CAD build for the part. Positions are in the model's coordinates, mm. A direction names the side the tool comes from. Give positions to 0.01 mm unless a question says otherwise; leave off trailing zeros. Loops run counter-clockwise (first coordinate to the right, second up) from the corner with the lowest first, then second, coordinate; pieces in that order, holes last. Notation, with made-up numbers: (-1.75, 24.5) - (19.25, 24.5) arc R32 cw to (19.25, 55.5) - close; hole circle Ø4 at (78, 49). An arc over 180 degrees is marked (long way). Return JSON: item names as keys, results as strings.
Autodesk Inventor part; units mm, degrees
ref_plane "YZ Plane" through (0, 0, 0) normal (1, 0, 0) x (0, 1, 0)
ref_plane "XZ Plane" through (0, 0, 0) normal (0, 1, 0) x (-1, 0, 0)
ref_plane "XY Plane" through (0, 0, 0) normal (0, 0, 1) x (1, 0, 0)
sketch "Sketch1" plane through (0, 0, 0) normal (0, 0, 1) x (1, 0, 0)
  line L0 (0, -9.7468) -> (0, 24.9578) construction
  line L1 (-29.249, 0) -> (29.249, 0) construction
  arc A0 (-18.0821, 3.4154) -> (-16, -4) centre (-16, 0) ccw
  line L2 (-16, -4) -> (16, -4)
  arc A1 (16, -4) -> (18.0821, 3.4154) centre (16, 0) ccw
  line L3 (-18.0821, 3.4154) -> (-4, 12)
  line L4 (-4, 12) -> (-4, 16)
  arc A2 (4, 16) -> (-4, 16) centre (0, 16) ccw
  line L5 (4, 16) -> (4, 12)
  line L6 (4, 12) -> (18.0821, 3.4154)
  point P0 (0, -4)
  dimension "d0" = 40
  dimension "d38" = 8
  dimension "d39" = 24
  dimension "d41" = 4
sketch "Sketch8" plane through (0, 0, 0) normal (0, 0, 1) x (1, 0, 0)
  circle A0 centre (0, 0) radius 2.4
  circle A1 centre (0, 0) radius 2.75
  circle A2 centre (0, 16) radius 2.4
  circle A3 centre (0, 16) radius 2.75
  arc A4 (4, 16) -> (-4, 16) centre (0, 16) ccw construction
  line L0 (0, 16) -> (0, 0) construction
  circle A5 centre (0, 8) radius 2.4
  circle A6 centre (0, 8) radius 2.75
  circle A7 centre (-8, 0) radius 2.4
  circle A8 centre (-8, 0) radius 2.75
  circle A9 centre (8, 0) radius 2.4
  circle A10 centre (8, 0) radius 2.75
  line L1 (-8, 0) -> (8, 0) construction
  dimension "d42" = 5.5
  dimension "d43" = 4.8
sketch "Sketch6" plane through (0, 0, 0) normal (0, 0, 1) x (1, 0, 0)
  arc A0 (-18.0821, 3.4154) -> (-16, -4) centre (-16, 0) ccw construction
  arc A1 (16, -4) -> (18.0821, 3.4154) centre (16, 0) ccw construction
  circle A2 centre (-16, 0) radius 2.3
  circle A3 centre (16, 0) radius 2.3
  line L0 (-18.1564, 0.8) -> (-16.8, 0.8)
  line L1 (-16.8, 0.8) -> (-16.8, 2.1564)
  line L2 (-15.2, 2.1564) -> (-15.2, 0.8)
  line L3 (-15.2, 0.8) -> (-13.8436, 0.8)
  line L4 (-13.8436, -0.8) -> (-15.2, -0.8)
  line L5 (-15.2, -0.8) -> (-15.2, -2.1564)
  line L6 (-16.8, -2.1564) -> (-16.8, -0.8)
  line L7 (-16.8, -0.8) -> (-18.1564, -0.8)
  line L8 (13.8436, 0.8) -> (15.2, 0.8)
  line L9 (16.8, 0.8) -> (18.1564, 0.8)
  line L10 (16.8, 2.1564) -> (16.8, 0.8)
  line L11 (16.8, -0.8) -> (16.8, -2.1564)
  line L12 (15.2, 2.1564) -> (15.2, 0.8)
  line L13 (15.2, -0.8) -> (15.2, -2.1564)
  line L14 (18.1564, -0.8) -> (16.8, -0.8)
  line L15 (15.2, -0.8) -> (13.8436, -0.8)
  circle A4 centre (-16, 0) radius 2.75
  circle A5 centre (16, 0) radius 2.75
  dimension "d29" = 4.6
  dimension "d30" = 1.6
  dimension "d44" = 5.5
extrude "Extrusion1" add sketch "Sketch1" along normal mid plane 4
extrude "Extrusion9" cut sketch "Sketch6" along normal through all both and the other way through all contours A2 L4 L5 L6 L7 L0 L1 L2 L3 | A3 L14 L11 L13 L15 L8 L12 L10 L9
extrude "Extrusion10" cut sketch "Sketch8" along normal through all both and the other way through all contours A0 | A2 | A5 | A7 | A9
sketch "Sketch2" plane through (0, 0, 2) normal (0, 0, 1) x (1, 0, 0)
  circle A0 centre (0, 0) radius 2.75
  circle A1 centre (-8, 0) radius 2.75
  circle A2 centre (0, 8) radius 2.75
  circle A3 centre (8, 0) radius 2.75
  circle A4 centre (0, 16) radius 2.75
extrude "Extrusion3" cut sketch "Sketch2" against normal blind 0.5333
sketch "Sketch3" plane through (0, 0, -2) normal (0, 0, -1) x (-1, 0, 0)
  circle A0 centre (0, 0) radius 2.75
  circle A1 centre (-8, 0) radius 2.75
  circle A2 centre (8, 0) radius 2.75
  circle A3 centre (0, 8) radius 2.75
  circle A4 centre (0, 16) radius 2.75
extrude "Extrusion4" cut sketch "Sketch3" against normal blind 0.5333
sketch "Sketch9" plane through (0, 0, 2) normal (0, 0, 1) x (1, 0, 0)
  circle A0 centre (0, 16) radius 2.75 construction
  circle A1 centre (0, 8) radius 2.75 construction
  line L0 (4, 12) -> (18.0821, 3.4154) construction
  line L1 (-18.0821, 3.4154) -> (-4, 12) construction
  circle A2 centre (-8, 0) radius 2.75 construction
  circle A3 centre (0, 0) radius 2.75 construction
  circle A4 centre (8, 0) radius 2.75 construction
  circle A5 centre (-16, 0) radius 2.75 construction
  circle A6 centre (16, 0) radius 2.75 construction
  line L2 (1.3037, 12.6027) -> (16.0078, 3.6389)
  arc A7 (16.0078, 3.6389) -> (14.1125, -3.1111) centre (16, 0) ccw
  line L3 (-16.0078, 3.6389) -> (-1.3037, 12.6027)
  arc A8 (-14.1125, -3.1111) -> (-16.0078, 3.6389) centre (-16, 0) ccw
  line L4 (-28, 0) -> (28, 0) construction
  line L5 (0, -8.8) -> (0, 24.8) construction
  line L6 (16, -4) -> (-16, -4) construction
  arc A9 (-6.1125, -3.1111) -> (-9.8875, -3.1111) centre (-8, 0) ccw
  line L7 (-14.1125, -3.1111) -> (-9.8875, -3.1111)
  line L8 (-6.1125, -3.1111) -> (-1.8875, -3.1111)
  arc A10 (1.8875, -3.1111) -> (-1.8875, -3.1111) centre (0, 0) ccw
  line L9 (1.8875, -3.1111) -> (6.1125, -3.1111)
  arc A11 (9.8875, -3.1111) -> (6.1125, -3.1111) centre (8, 0) ccw
  line L10 (9.8875, -3.1111) -> (14.1125, -3.1111)
  arc A12 (-3.1111, 14.1125) -> (3.1111, 14.1125) centre (0, 16) ccw
  arc A13 (3.1111, 9.8875) -> (-3.1111, 9.8875) centre (0, 8) ccw
  line L11 (-3.1111, 14.1125) -> (-3.1111, 9.8875)
  line L12 (3.1111, 14.1125) -> (3.1111, 9.8875)
  line L13 (-4, 12) -> (-4, 16) construction
  line L14 (4, 16) -> (4, 12) construction
  arc A14 (-0.6774, 11.5753) -> (0.6774, 11.5753) centre (0, 8) ccw
  line L15 (1.3037, 12.6027) -> (0.6774, 11.5753)
  line L16 (-1.3037, 12.6027) -> (-0.6774, 11.5753)
  dimension "d52" = 0.8889
  dimension "d53" = 0.8889
  dimension "d54" = 0.8889
  dimension "d55" = 0.8889
  dimension "d58" = 0.8889
  dimension "d59" = 0.8889
extrude "Extrusion11" cut sketch "Sketch9" against normal blind 0.5333 contours A12 L12 L2 | L15 A13 L16 A12 | L2 L12 A13 L15 | L2 A7 L10 A11 L9 A10 L8 A9 L7 A8 L3 L11 A14 L12 | L16 A13 L11 L3 | L3 L11 A12
sketch "Sketch10" plane through (0, 0, -2) normal (0, 0, -1) x (-1, 0, 0)
  arc A0 (-3.1111, 14.1125) -> (3.1111, 14.1125) centre (0, 16) ccw
  line L0 (3.1111, 14.1125) -> (3.1111, 11.5008)
  line L1 (3.1111, 11.5008) -> (16.0078, 3.6389)
  arc A1 (16.0078, 3.6389) -> (14.1125, -3.1111) centre (16, 0) ccw
  line L2 (14.1125, -3.1111) -> (9.8875, -3.1111)
  arc A2 (9.8875, -3.1111) -> (6.1125, -3.1111) centre (8, 0) ccw
  line L3 (6.1125, -3.1111) -> (1.8875, -3.1111)
  arc A3 (1.8875, -3.1111) -> (-1.8875, -3.1111) centre (0, 0) ccw
  line L4 (-1.8875, -3.1111) -> (-6.1125, -3.1111)
  arc A4 (-6.1125, -3.1111) -> (-9.8875, -3.1111) centre (-8, 0) ccw
  line L5 (-9.8875, -3.1111) -> (-14.1125, -3.1111)
  arc A5 (-14.1125, -3.1111) -> (-16.0078, 3.6389) centre (-16, 0) ccw
  line L6 (-16.0078, 3.6389) -> (-3.1111, 11.5008)
  line L7 (-3.1111, 11.5008) -> (-3.1111, 14.1125)
  circle A6 centre (0, 8) radius 3.6389
extrude "Extrusion12" cut sketch "Sketch10" against normal blind 0.5333
equation "\"d38\" = width_standard"
equation "\"d41\" = 0.5 * width_standard"
equation "\"d2\" = 0.5 * width_standard"
equation "\"d13\" = 0.0555556 * height_standard"
equation "\"d15\" = 0.0555556 * height_standard"
equation "\"d56\" = 0.0555556 * height_standard"
equation "\"d60\" = 0.0555556 * height_standard"
equation "\"width_standard\" = 8"
equation "\"height_standard\" = 9.6"
properties part number "LEGO Brick 32017" material "Steel"
1. Which spindle directions (+Z, -Z, +X, -X, +Y, -Y) get a long thin tool onto all of the face, cutting with end or side? Do faces 4 (the face through (17, -0.8, 0)), 5 (the face through (0, 4, 1.467)), 6 (the face through (4, 14, 0)). Say none if no direction does.
Values follow:
{"face 4": "+Z, -Z", "face 5": "+Z", "face 6": "+Z, -Z, +X, +Y"}
2. Cut at C-C, the plane z = -0.1. Give the number of separate pieces and of enclosed holes in the cut face, plus the area to 3 significant figures.
Values follow:
{"separate pieces": "1", "enclosed holes": "7", "area": "418 mm²"}
3. Drop flat-ended pins along their axis: P1, Ø2, axis at x = 12, z = 0.5, coming from the +Y side; P2, Ø2, axis at y = 14.5, z = -0.5, coming from the -X side; P3, Ø0.6, axis at x = -3, z = -1.5, coming from the +Y side. Give the stop position or say it passes through.
Values follow:
{"P1": "stops at y = 7.73", "P2": "stops at x = -4", "P3": "stops at y = 18.95"}
4. Pull direction X, two halves, no side cores. Call faces 1 (the face through (-1.6, 2.7, -2)), 2 (the face through (-11.14, 7.648, -0.028)), 3 (the face through (10.54, -1.05, 1.74)): +X half, -X half, draft (parallel to the pull), parting line (faces both ways), or undercut.
Values follow:
{"face 1": "draft", "face 2": "-X half", "face 3": "undercut"}
5. Cut at A-A, the plane x = 8. Write the cut outline in (y, z).
Values follow:
{"outline": "(-4, -2) - (-2.75, -2) - (-2.75, -1.47) - (-2.4, -1.47) - (-2.4, 1.47) - (-2.75, 1.47) - (-2.75, 2) - (-4, 2) - close; (2.4, -1.47) - (2.75, -1.47) - (2.75, -2) - (3.64, -2) - (3.64, -1.47) - (8.52, -1.47) - (8.52, -2) - (9.56, -2) - (9.56, 2) - (8.52, 2) - (8.52, 1.47) - (3.64, 1.47) - (3.64, 2) - (2.75, 2) - (2.75, 1.47) - (2.4, 1.47) - close"}
6. Cut at B-B, the plane y = 17. Write the cut outline in (x, z), plus the area to 3 significant figures.
Values follow:
{"outline": "(-3.87, -2) - (-2.56, -2) - (-2.56, -1.47) - (-2.18, -1.47) - (-2.18, 1.47) - (-2.56, 1.47) - (-2.56, 2) - (-3.87, 2) - close; (2.18, -1.47) - (2.56, -1.47) - (2.56, -2) - (3.87, -2) - (3.87, 2) - (2.56, 2) - (2.56, 1.47) - (2.18, 1.47) - close", "area": "12.7 mm²"}
7. Drill centre lines: probe 1 along Y at (x, z) = (-8, 1.75); probe 2 along Y at (x, z) = (-2, 0.6); probe 3 along X at (y, z) = (12.25, -0.95). Where is each one in solid material? Low to high.
Values follow:
{"probe 1": "y = -4 to -2.75, 2.75 to 3.64, 8.52 to 9.56", "probe 2": "y = -4 to -1.33, 1.33 to 6.67, 9.33 to 14.67, 17.33 to 19.46", "probe 3": "x = -4 to 4"}
